from build123d import *

# Parameters (mm, degrees)
BOX179_W                     = 56
BOX179_H                     = 200
BOX179_DEPTH                 = 47
CYLINDER2007_R               = 1.5
CYLINDER2007_DEPTH           = 72
CYLINDER2007_PLACEMENT_ANGLE = 30
CYLINDER2006_R               = 1.5
CYLINDER2006_DEPTH           = 72
CYLINDER2006_PLACEMENT_ANGLE = 60
CYLINDER2011_R               = 1.5
CYLINDER2011_DEPTH           = 72
CYLINDER2012_R               = 1.5
CYLINDER2012_DEPTH           = 72
CYLINDER2012_PLACEMENT_ANGLE = 120
CYLINDER2013_R               = 1.5
CYLINDER2013_DEPTH           = 72
CYLINDER2013_PLACEMENT_ANGLE = 150
CYLINDER2010_R               = 1.5
CYLINDER2010_DEPTH           = 72
CYLINDER2017_R               = 1.5
CYLINDER2017_DEPTH           = 72
CYLINDER2017_PLACEMENT_ANGLE = 210
CYLINDER2016_R               = 1.5
CYLINDER2016_DEPTH           = 72
CYLINDER2016_PLACEMENT_ANGLE = 240
CYLINDER2015_R               = 1.5
CYLINDER2015_DEPTH           = 72
CYLINDER2008_R               = 1.5
CYLINDER2008_DEPTH           = 72
CYLINDER2008_PLACEMENT_ANGLE = 60
CYLINDER2014_R               = 1.5
CYLINDER2014_DEPTH           = 72
CYLINDER2014_PLACEMENT_ANGLE = 30
CYLINDER2009_R               = 1.5
CYLINDER2009_DEPTH           = 72
TUBE052_R                    = 74
TUBE052_R_2                  = 60
TUBE052_DEPTH                = 4


with BuildPart() as krychle179:
    # Box179 → Box179 (new body)
    with BuildSketch(Plane(origin=(-28, 0, 27), x_dir=(1, 0, 0), z_dir=(0, 0, 1))):
        with Locations((28, 100)):
            Rectangle(BOX179_W, BOX179_H)
    extrude(amount=BOX179_DEPTH)


with BuildPart() as obj1:
    # Cylinder2007 → Cylinder2007 (new body)
    with BuildSketch(Plane.XY):
        Circle(CYLINDER2007_R)
    extrude(amount=CYLINDER2007_DEPTH)


with BuildPart() as obj1_1:
    # Cylinder2007 placement: moved
    add(obj1.part.moved(Location((35.5, -61.487804, 0))).rotate(Axis((35.5, -61.487804, 0), (0, 0, 1)), CYLINDER2007_PLACEMENT_ANGLE))


with BuildPart() as obj2:
    # Cylinder2006 → Cylinder2006 (new body)
    with BuildSketch(Plane.XY):
        Circle(CYLINDER2006_R)
    extrude(amount=CYLINDER2006_DEPTH)


with BuildPart() as obj2_1:
    # Cylinder2006 placement: moved
    add(obj2.part.moved(Location((61.487804, -35.5, 0))).rotate(Axis((61.487804, -35.5, 0), (0, 0, 1)), CYLINDER2006_PLACEMENT_ANGLE))


with BuildPart() as obj3:
    # Cylinder2011 → Cylinder2011 (new body)
    with BuildSketch(Plane(origin=(71, 0, 0), x_dir=(0, 1, 0), z_dir=(0, 0, 1))):
        Circle(CYLINDER2011_R)
    extrude(amount=CYLINDER2011_DEPTH)


with BuildPart() as obj4:
    # Cylinder2012 → Cylinder2012 (new body)
    with BuildSketch(Plane.XY):
        Circle(CYLINDER2012_R)
    extrude(amount=CYLINDER2012_DEPTH)


with BuildPart() as obj4_1:
    # Cylinder2012 placement: moved
    add(obj4.part.moved(Location((61.487804, 35.5, 0))).rotate(Axis((61.487804, 35.5, 0), (0, 0, 1)), CYLINDER2012_PLACEMENT_ANGLE))


with BuildPart() as obj5:
    # Cylinder2013 → Cylinder2013 (new body)
    with BuildSketch(Plane.XY):
        Circle(CYLINDER2013_R)
    extrude(amount=CYLINDER2013_DEPTH)


with BuildPart() as obj5_1:
    # Cylinder2013 placement: moved
    add(obj5.part.moved(Location((35.5, 61.487804, 0))).rotate(Axis((35.5, 61.487804, 0), (0, 0, 1)), CYLINDER2013_PLACEMENT_ANGLE))


with BuildPart() as obj6:
    # Cylinder2010 → Cylinder2010 (new body)
    with BuildSketch(Plane(origin=(0, 71, 0), x_dir=(-1, 0, 0), z_dir=(0, 0, 1))):
        Circle(CYLINDER2010_R)
    extrude(amount=CYLINDER2010_DEPTH)


with BuildPart() as obj7:
    # Cylinder2017 → Cylinder2017 (new body)
    with BuildSketch(Plane.XY):
        Circle(CYLINDER2017_R)
    extrude(amount=CYLINDER2017_DEPTH)


with BuildPart() as obj7_1:
    # Cylinder2017 placement: moved
    add(obj7.part.moved(Location((-35.5, 61.487804, 0))).rotate(Axis((-35.5, 61.487804, 0), (0, 0, 1)), CYLINDER2017_PLACEMENT_ANGLE))


with BuildPart() as obj8:
    # Cylinder2016 → Cylinder2016 (new body)
    with BuildSketch(Plane.XY):
        Circle(CYLINDER2016_R)
    extrude(amount=CYLINDER2016_DEPTH)


with BuildPart() as obj8_1:
    # Cylinder2016 placement: moved
    add(obj8.part.moved(Location((-61.487804, 35.5, 0))).rotate(Axis((-61.487804, 35.5, 0), (0, 0, 1)), CYLINDER2016_PLACEMENT_ANGLE))


with BuildPart() as obj9:
    # Cylinder2015 → Cylinder2015 (new body)
    with BuildSketch(Plane(origin=(-71, 0, 0), x_dir=(0, -1, 0), z_dir=(0, 0, 1))):
        Circle(CYLINDER2015_R)
    extrude(amount=CYLINDER2015_DEPTH)


with BuildPart() as obj10:
    # Cylinder2008 → Cylinder2008 (new body)
    with BuildSketch(Plane.XY):
        Circle(CYLINDER2008_R)
    extrude(amount=CYLINDER2008_DEPTH)


with BuildPart() as obj10_1:
    # Cylinder2008 placement: moved
    add(obj10.part.moved(Location((-61.487804, -35.5, 0))).rotate(Axis((-61.487804, -35.5, 0), (0, 0, -1)), CYLINDER2008_PLACEMENT_ANGLE))


with BuildPart() as obj11:
    # Cylinder2014 → Cylinder2014 (new body)
    with BuildSketch(Plane.XY):
        Circle(CYLINDER2014_R)
    extrude(amount=CYLINDER2014_DEPTH)


with BuildPart() as obj11_1:
    # Cylinder2014 placement: moved
    add(obj11.part.moved(Location((-35.5, -61.487804, 0))).rotate(Axis((-35.5, -61.487804, 0), (0, 0, -1)), CYLINDER2014_PLACEMENT_ANGLE))


with BuildPart() as compound1084:
    # Cylinder2009 → Cylinder2009 (new body)
    with BuildSketch(Plane(origin=(0, -71, 0), x_dir=(1, 0, 0), z_dir=(0, 0, 1))):
        Circle(CYLINDER2009_R)
    extrude(amount=CYLINDER2009_DEPTH)

    # Compound1084: union obj1, obj2, obj3, obj4, obj5, obj6, obj7, obj8, obj9, obj10, obj11
    add(obj1_1.part)
    add(obj2_1.part)
    add(obj3.part)
    add(obj4_1.part)
    add(obj5_1.part)
    add(obj6.part)
    add(obj7_1.part)
    add(obj8_1.part)
    add(obj9.part)
    add(obj10_1.part)
    add(obj11_1.part)


with BuildPart() as compound1084_1:
    # Compound1084 placement: moved
    add(compound1084.part.moved(Location((0, 0, -4))))


with BuildPart() as cut683:
    # Tube052 → Tube052 (new body)
    with BuildSketch(Plane.XY.offset(25)):
        Circle(TUBE052_R)
        Circle(TUBE052_R_2, mode=Mode.SUBTRACT)
    extrude(amount=TUBE052_DEPTH)

    # Cut678: cut Compound1084
    add(compound1084_1.part, mode=Mode.SUBTRACT)

    # Cut683: cut Krychle179
    add(krychle179.part, mode=Mode.SUBTRACT)


solid = cut683.part
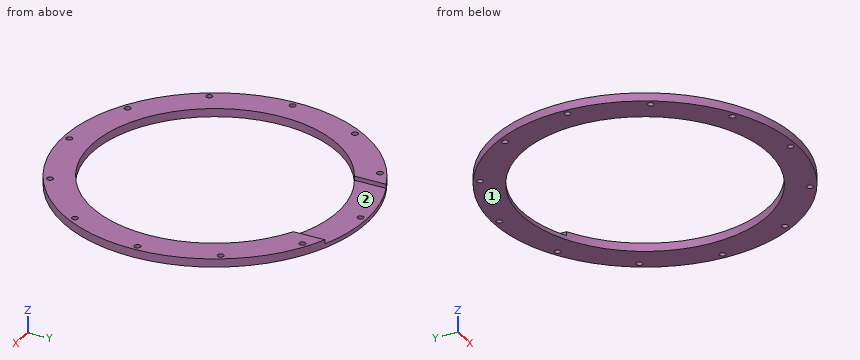
Check sheet for the modelled part. Datum: model origin and axes. Units: mm. Face numbers are marked on the shaded views. Round coordinates to 2 decimals unless told otherwise and drop trailing zeros. Write each loop counter-clockwise with the first axis right and the second up, starting at its lowest first coordinate (ties: lowest second). Pieces come first, ordered by that corner, then holes. Notation, with made-up numbers: (-20, 54.25) -> (2, 54.25) arc R15 cw to (2, 59.25) -> close; hole circle Ø6 at (16.25, 58). An arc over 180 degrees is marked (long way). Answer as CSV lines item,"result". Start each with the question number.
1) Release check for a two-part mould opening along X. For the marked faces 1 and 2 record: pulls with the +X half, pulls with the -X half, needs draft (parallel to the pull), parting line crosses it, or undercut.
2) Section check C-C on x = -31.5. Enter the section's corners in (y, z).
3) Section check A-A on z = 28. State how many separate pieces and enclosed holes the cut face has, and give its area (3 significant figures).
4) Material ranges on line 1 (Y direction, x = 0, z = 25.8); line 2 (X direction, y = -2, z = 26.3), recorded low to high. Write a range as from..to.
5) Section check B-B on y = -49.5. Enter the section's corners in (x, z), and give its area (3 significant figures).
6) Go/stop test with flat-tipped pins: P1, Ø2.5, axis at x = -61.49, y = -35.5, coming from the +Z side; P2, Ø10.5, axis at x = -13, y = 64.5, coming from the +Z side; P3, Ø1, axis at y = 11, z = 26, coming from the -X side; P4, Ø1, axis at x = 6.5, z = 27, coming from the -Y side. Record where each tip stops, or that it passes through.
Found:
1,face 1,"needs draft"
1,face 2,"undercut"
2,outline,"(-66.96, 25) -> (-51.07, 25) -> (-51.07, 29) -> (-66.96, 29) -> close; (51.07, 25) -> (66.96, 25) -> (66.96, 29) -> (51.07, 29) -> close"
3,separate pieces,"1"
3,enclosed holes,"11"
3,area,"5,010 mm^2"
4,line 1,"y = -74..-72.5, -69.5..-60, 60..69.5, 72.5..74"
4,line 2,"x = -73.97..-59.97, 59.97..73.97"
5,outline,"(-55.01, 25) -> (-33.91, 25) -> (-33.91, 29) -> (-55.01, 29) -> close; (33.91, 25) -> (55.01, 25) -> (55.01, 29) -> (33.91, 29) -> close"
5,area,"169 mm^2"
6,P1,"passes through"
6,P2,"stops at z = 27"
6,P3,"stops at x = -73.25"
6,P4,"stops at y = -73.76"
